Geometry: see drawing. Coordinates: mm, zero at the bounding-box minimum. A direction names the side the tool comes from. Coordinates: 2 decimals unless noted, no trailing zeros. Loops run counter-clockwise (first coordinate to the right, second up) from the corner with the lowest first, then second, coordinate; pieces in that order, holes last. Notation, with made-up numbers: M -15,81.5 L 22,81.5 A21 ccw 22,118.5 Z; hole C -40,14 d10. An arc over 180 degrees is marked long. Write each question's results on one line, items separated by ' | '. Start each with the question number.
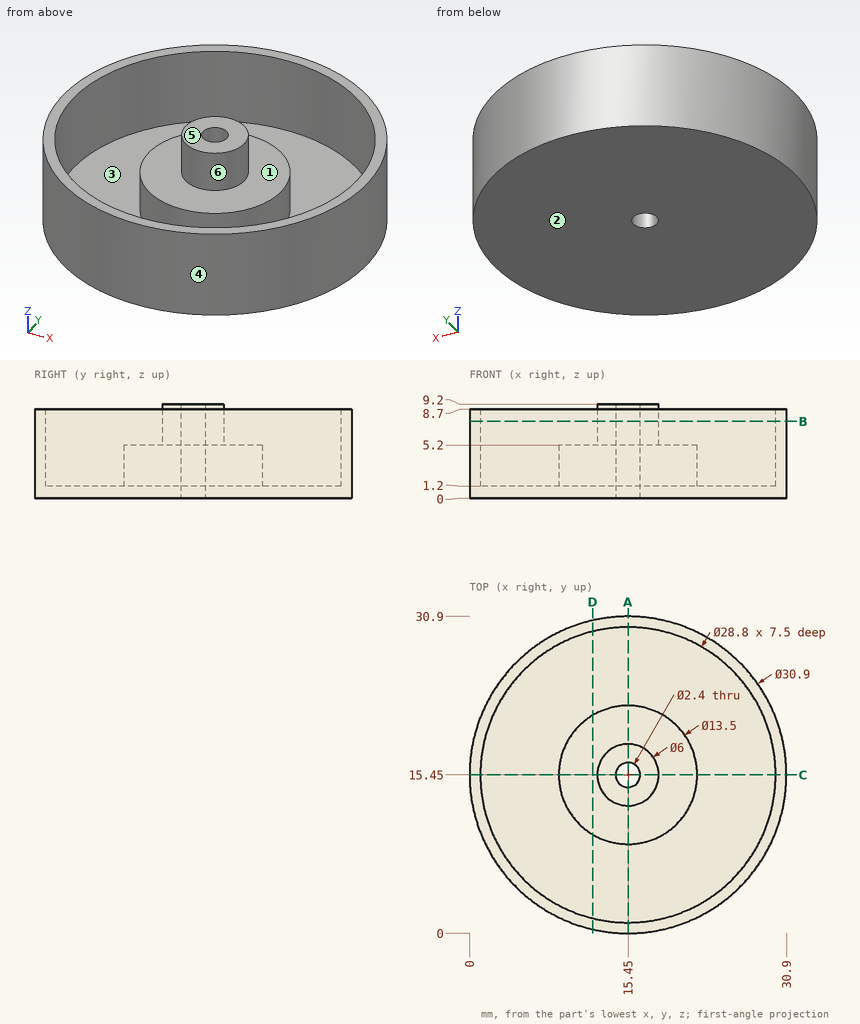
Item 1: Line query: probe 1 along Y at (x, z) = (15.45, 5.25); probe 2 along Y at (x, z) = (15.45, 3.5); probe 3 along X at (y, z) = (17, 2.25). Output: solid intervals per line, ascending.
Item 2: Cut plane D-D (x = 12). Output: boundary loops of the cut face in (y, z).
Item 3: Access query for the marked faces 5 and 6. Directions: +Z, -Z, +X, -X, +Y, -Y. A direction counts if a zero-diameter tool reaches every point of the face in a straight line with its end or side. Return the directions, or none.
Item 4: Mould query, pull axis Y, two halves, no side actions, for the marked faces 1, 2, 3 and 4. Classes: +Y half, -Y half, draft (parallel to the pull), parting line (faces both ways), or undercut.
Item 5: Cut plane A-A (x = 15.45). Output: boundary loops of the cut face in (y, z), then the cut area to 3 significant figures.
Item 6: Cut plane B-B (z = 7.5). Output: boundary loops of the cut face in (x, y).
Item 7: First-contact query: pin 1 Ø6 at (x, y) = (23, 14.5) entering from +Z; pin 2 Ø4 at (x, z) = (5, 6.5) entering from -Y; pin 3 Ø1.9 at (x, y) = (15.45, 15.45) entering from -Z; pin 4 Ø12 at (x, y) = (25.5, 18.5) entering from +Z. Flat tips, straight axial feed; report the tip coordinate or a pass-through.
Response values:
1) probe 1: y = 0 to 1.05, 12.45 to 14.25, 16.65 to 18.45, 29.85 to 30.9 | probe 2: y = 0 to 1.05, 8.7 to 14.25, 16.65 to 22.2, 29.85 to 30.9 | probe 3: x = 0.08 to 1.13, 8.88 to 22.02, 29.77 to 30.82
2) outline: M 0.39,0 L 30.51,0 L 30.51,8.7 L 29.43,8.7 L 29.43,1.2 L 21.25,1.2 L 21.25,5.2 L 9.65,5.2 L 9.65,1.2 L 1.47,1.2 L 1.47,8.7 L 0.39,8.7 Z
3) face 5: +Z, +X, -X, +Y, -Y | face 6: +Z
4) face 1: undercut | face 2: draft | face 3: undercut | face 4: parting line
5) outline: M 0,0 L 14.25,0 L 14.25,9.2 L 12.45,9.2 L 12.45,5.2 L 8.7,5.2 L 8.7,1.2 L 1.05,1.2 L 1.05,8.7 L 0,8.7 Z; M 16.65,0 L 30.9,0 L 30.9,8.7 L 29.85,8.7 L 29.85,1.2 L 22.2,1.2 L 22.2,5.2 L 18.45,5.2 L 18.45,9.2 L 16.65,9.2 Z | area: 109 mm2
6) outline: C 15.45,15.45 d30.9; C 15.45,15.45 d6; hole C 15.45,15.45 d28.8; hole C 15.45,15.45 d2.4
7) pin 1: stops at z = 5.2 | pin 2: stops at y = 2.52 | pin 3: passes through | pin 4: stops at z = 8.7
